from build123d import *

# Parameters (mm, degrees)
EXTRUDE_1_DEPTH        = 3.85
SKETCH_2_R             = 1.1
CUT_EXTRUDE_1_DEPTH    = 4.85
CUT_EXTRUDE_2_DEPTH    = 2.1
PATTERN_LINEAR_1_COUNT = 2
PATTERN_LINEAR_1_PITCH = 40
PATTERN_LINEAR_2_COUNT = 2
PATTERN_LINEAR_2_PITCH = 40
SKETCH_7_R             = 2.5
SKETCH_7_R_2           = 1.1
EXTRUDE_2_DEPTH        = 2.6
SKETCH_8_R             = 2.65
CUT_EXTRUDE_5_DEPTH    = 2
SKETCH_5_W             = 17
SKETCH_5_H             = 23
CUT_EXTRUDE_3_DEPTH    = 1.85
SKETCH_6_R             = 4
CUT_EXTRUDE_4_DEPTH    = 1.85
SKETCH_9_W             = 24
SKETCH_9_H             = 67
CUT_EXTRUDE_6_DEPTH    = 0.85
SKETCH_10_R            = 3
CUT_EXTRUDE_7_DEPTH    = 2.65
SKETCH_11_R            = 4.5
CUT_EXTRUDE_8_DEPTH    = 2.85


with BuildPart() as part:
    # 草图1 → 凸台-拉伸1 (new body)
    with BuildSketch(Plane(origin=(0, 0, 0), x_dir=(1, 0, 0), z_dir=(0, 1, 0))):
        with BuildLine():
            Line((-52.9, -45.9), (52.9, -45.9))
            ThreePointArc((52.9, -45.9), (54.314213562, -45.314213562), (54.9, -43.9))
            Line((54.9, -43.9), (54.9, 43.9))
            ThreePointArc((54.9, 43.9), (54.314213562, 45.314213562), (52.9, 45.9))
            Line((52.9, 45.9), (-52.9, 45.9))
            ThreePointArc((-52.9, 45.9), (-54.314213562, 45.314213562), (-54.9, 43.9))
            Line((-54.9, 43.9), (-54.9, -43.9))
            ThreePointArc((-54.9, -43.9), (-54.314213562, -45.314213562), (-52.9, -45.9))
        make_face()
    extrude(amount=EXTRUDE_1_DEPTH)

    # 草图2 → 切除-拉伸1 (cut, through all)
    with BuildSketch(Plane(origin=(0, 3.85, 0), x_dir=(1, 0, 0), z_dir=(0, 1, 0))):
        with Locations((-40.5, 37.25)):
            Circle(SKETCH_2_R)
        with Locations((51.5, 37.25)):
            Circle(SKETCH_2_R)
    extrude(amount=-CUT_EXTRUDE_1_DEPTH, mode=Mode.SUBTRACT)

    # 草图3 → 切除-拉伸2 (cut, symmetric)
    with BuildSketch(Plane(origin=(0, 0, 0), x_dir=(0, 0, -1), z_dir=(1, 0, 0))):
        Polygon((-45.9, 3.85), (-43.3, 3.85), (-43.3, 2.922792206), (-44.572792206, 1.65), (-45.9, 1.65), align=None)
    cut_extrude_2 = extrude(amount=CUT_EXTRUDE_2_DEPTH, both=True, mode=Mode.SUBTRACT)

    # 阵列(线性)1: 切除-拉伸2 ×2
    with Locations(*[(i * PATTERN_LINEAR_1_PITCH, 0, 0) for i in range(1, PATTERN_LINEAR_1_COUNT)]):
        add(cut_extrude_2, mode=Mode.SUBTRACT)

    # 阵列(线性)2: 切除-拉伸2 ×2
    with Locations(*[(-i * PATTERN_LINEAR_2_PITCH, 0, 0) for i in range(1, PATTERN_LINEAR_2_COUNT)]):
        add(cut_extrude_2, mode=Mode.SUBTRACT)

    # 草图7 → 凸台-拉伸2 (add)
    with BuildSketch(Plane.XZ):
        with Locations((-40.5, -37.25)):
            Circle(SKETCH_7_R)
        with Locations((-40.5, -37.25)):
            Circle(SKETCH_7_R_2, mode=Mode.SUBTRACT)
        with Locations((51.5, -37.25)):
            Circle(SKETCH_7_R)
        with Locations((51.5, -37.25)):
            Circle(SKETCH_7_R_2, mode=Mode.SUBTRACT)
        with Locations((-11.5, 19.75)):
            Circle(SKETCH_7_R)
        with Locations((-22.5, -14.25)):
            Circle(SKETCH_7_R)
        with Locations((12.5, 8.75)):
            Circle(SKETCH_7_R)
        with BuildLine():
            Line((-28.5, 40.9), (-1.5, 40.9))
            ThreePointArc((-1.5, 40.9), (0.5, 38.9), (-1.5, 36.9))
            Line((-1.5, 36.9), (-28.5, 36.9))
            ThreePointArc((-28.5, 36.9), (-30.5, 38.9), (-28.5, 40.9))
        make_face()
        with BuildLine():
            Line((47.5, 28.75), (47.5, 6.75))
            ThreePointArc((47.5, 6.75), (45.5, 4.75), (43.5, 6.75))
            Line((43.5, 6.75), (43.5, 28.75))
            ThreePointArc((43.5, 28.75), (45.5, 30.75), (47.5, 28.75))
        make_face()
        with BuildLine():
            Line((-7.5, -35.75), (42.5, -35.75))
            ThreePointArc((42.5, -35.75), (44.5, -37.75), (42.5, -39.75))
            Line((42.5, -39.75), (-7.5, -39.75))
            ThreePointArc((-7.5, -39.75), (-9.5, -37.75), (-7.5, -35.75))
        make_face()
    extrude(amount=EXTRUDE_2_DEPTH)

    # 草图8 → 切除-拉伸5 (cut)
    with BuildSketch(Plane(origin=(0, 3.85, 0), x_dir=(1, 0, 0), z_dir=(0, 1, 0))):
        with Locations((-40.5, 37.25)):
            Circle(SKETCH_8_R)
        with Locations((51.5, 37.25)):
            Circle(SKETCH_8_R)
    extrude(amount=-CUT_EXTRUDE_5_DEPTH, mode=Mode.SUBTRACT)

    # 草图5 → 切除-拉伸3 (cut)
    with BuildSketch(Plane.XZ):
        with Locations((28, 32.25)):
            Rectangle(SKETCH_5_W, SKETCH_5_H)
    extrude(amount=-CUT_EXTRUDE_3_DEPTH, mode=Mode.SUBTRACT)

    # 草图6 → 切除-拉伸4 (cut)
    with BuildSketch(Plane.XZ):
        with Locations((46.5, 0.75)):
            Circle(SKETCH_6_R)
    extrude(amount=-CUT_EXTRUDE_4_DEPTH, mode=Mode.SUBTRACT)

    # 草图9 → 切除-拉伸6 (cut)
    with BuildSketch(Plane.XZ):
        with Locations((-42.9, 12.4)):
            Rectangle(SKETCH_9_W, SKETCH_9_H)
    extrude(amount=-CUT_EXTRUDE_6_DEPTH, mode=Mode.SUBTRACT)

    # 草图10 → 切除-拉伸7 (cut)
    with BuildSketch(Plane.XZ):
        with Locations((-37.4, 11.75)):
            Circle(SKETCH_10_R)
        with Locations((-37.4, -16.75)):
            Circle(SKETCH_10_R)
    extrude(amount=-CUT_EXTRUDE_7_DEPTH, mode=Mode.SUBTRACT)

    # 草图11 → 切除-拉伸8 (cut)
    with BuildSketch(Plane.XZ):
        with Locations((-26.5, 6.75)):
            Circle(SKETCH_11_R)
    extrude(amount=-CUT_EXTRUDE_8_DEPTH, mode=Mode.SUBTRACT)


solid = part.part
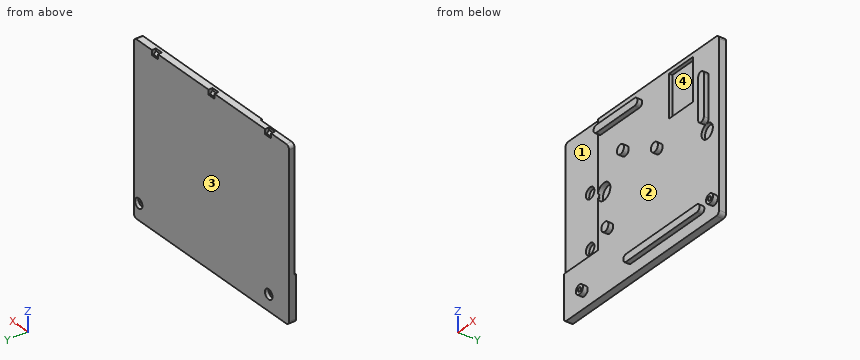
Source: CAD feature listing. Evaluate the final solid. Frame: model axes, mm. Face numbers are marked on the shaded views. A direction names the side the tool comes from. Coordinates: 2 decimals unless noted, no trailing zeros. Loops run counter-clockwise (first coordinate to the right, second up) from the corner with the lowest first, then second, coordinate; pieces in that order, holes last. Notation, with made-up numbers: (60, 52.25) - (67, 52.25) arc R24 cw to (67, 88.25) - close; hole circle Ø7 at (21.5, 64). An arc over 180 degrees is marked (long way). One line per item, written item: value. Start each with the question number.
1. Section B-B (x = -26.5). Return the cut outline in (y, z).
2. Section C-C (z = 25). Return the cut outline in (x, y), and give its area (3 significant figures).
3. Section D-D (z = 38.9). Return the cut outline in (x, y), and give its area (3 significant figures).
4. Contact query for flat-ended pins moving along their axis: P1, Ø1.3, axis at y = -2, z = 15, coming from the +X side; P2, Ø4, axis at x = -40.5, z = -37, coming from the +Y side; P3, Ø0.5, axis at x = 39.5, y = 3.5, coming from the +Z side. Output: stop coordinate, or through.
5. Mould query, pull axis X, two halves, no side actions, for the marked faces 3 and 4. Classes: pulls with the +X half, pulls with the -X half, needs draft (parallel to the pull), parting line crosses it, or undercut.
6. Set-up query: the marked faces 1 and 2. Return all of +Z, -Z, +X, -X, +Y, -Y with unobstructed straight access to the full face (end or side cutting, diameter ignored); none if empty.
7. Ray query, L1, parallel to Z at x = -37.4, y = 2.1; L2, parallel to Z at x = 46.5, y = 0.65; L3, parallel to Z at x = -40.5, y = 3.3. Return the intervals inside material, ascending.
8. Section A-A (y = -1). State how many separate pieces and enclosed holes the cut face has, and give its area (3 significant figures).
Verdict:
1. outline: (-2.6, 36.9) - (0, 36.9) - (0, 11.25) - (2.85, 11.25) - (2.85, 2.25) - (0, 2.25) - (0, -45.9) - (3.85, -45.9) - (3.85, 45.9) - (0, 45.9) - (0, 40.9) - (-2.6, 40.9) - close
2. outline: (-54.9, 0.85) - (-30.9, 0.85) - (-30.9, 0) - (19.5, 0) - (19.5, 1.85) - (36.5, 1.85) - (36.5, 0) - (43.5, 0) - (43.5, -2.6) - (47.5, -2.6) - (47.5, 0) - (54.9, 0) - (54.9, 3.85) - (-54.9, 3.85) - close
2. area: 381 mm2
3. outline: (-54.9, 0.85) - (-30.9, 0.85) - (-30.9, 0) - (-30.5, 0) - (-30.5, -2.6) - (0.5, -2.6) - (0.5, 0) - (19.5, 0) - (19.5, 1.85) - (36.5, 1.85) - (36.5, 0) - (54.9, 0) - (54.9, 3.85) - (-54.9, 3.85) - close
3. area: 451 mm2
4. P1: stops at x = 47.5
4. P2: stops at y = 1.85
4. P3: stops at z = 43.3
5. face 3: needs draft
5. face 4: undercut
6. face 1: +Z, -X, -Y
6. face 2: -Y
7. L1: z = -45.9 to -19.75, -13.75 to 8.75, 14.75 to 45.9
7. L2: z = -45.9 to -3.25, 4.75 to 45.9
7. L3: z = -45.9 to -39.9, -34.6 to 43.3
8. separate pieces: 8
8. enclosed holes: 2
8. area: 524 mm2
